from build123d import *

# Parameters (mm, degrees)
SKETCH1_W      = 6.35
SKETCH1_H      = 3.175
SKETCH1_W_2    = 12.7
SKETCH1_H_2    = 25
EXTRUDE1_DEPTH = 6.35


with BuildPart() as part:
    # Sketch1 → Extrude1 (new body)
    with BuildSketch(Plane.XY):
        with BuildLine():
            Line((-155, 0), (-155, 4))
            Line((-155, 4), (-180, 4))
            Line((-180, 4), (-180, 0))
            Line((-180, 0), (-195, 0))
            Line((-195, 0), (-179.241666667, 60))
            Line((-179.241666667, 60), (-146.84375, 60))
            Line((-146.84375, 60), (-146.84375, 85))
            Line((-146.84375, 85), (-172.675694444, 85))
            Line((-172.675694444, 85), (-166.109722222, 110))
            Line((-166.109722222, 110), (-146.84375, 110))
            Line((-146.84375, 110), (-146.84375, 135))
            Line((-146.84375, 135), (-159.54375, 135))
            Line((-159.54375, 135), (-152.977777778, 160))
            Line((-152.977777778, 160), (-134.14375, 160))
            ThreePointArc((-134.14375, 160), (-129.14375, 155), (-124.14375, 160))
            Line((-124.14375, 160), (-124.14375, 135))
            Line((-124.14375, 135), (-111.44375, 135))
            Line((-111.44375, 135), (-111.44375, 160))
            Line((-111.44375, 160), (0, 160))
            Line((0, 160), (124.14375, 160))
            ThreePointArc((124.14375, 160), (129.14375, 155), (134.14375, 160))
            Line((134.14375, 160), (152.977777778, 160))
            Line((152.977777778, 160), (159.54375, 135))
            Line((159.54375, 135), (111.44375, 135))
            Line((111.44375, 135), (111.44375, 110))
            Line((111.44375, 110), (166.109722222, 110))
            Line((166.109722222, 110), (172.675694444, 85))
            Line((172.675694444, 85), (111.44375, 85))
            Line((111.44375, 85), (111.44375, 60))
            Line((111.44375, 60), (179.241666667, 60))
            Line((179.241666667, 60), (195, 0))
            Line((195, 0), (180, 0))
            Line((180, 0), (180, 4))
            Line((180, 4), (155, 4))
            Line((155, 4), (155, 0))
            Line((155, 0), (-111.44375, 0))
            Line((-111.44375, 0), (-111.44375, 60))
            Line((-111.44375, 60), (-124.14375, 60))
            Line((-124.14375, 60), (-124.14375, 0))
            Line((-124.14375, 0), (-155, 0))
        make_face()
        with Locations((-53.175, 143.4125)):
            Rectangle(SKETCH1_W, SKETCH1_H, mode=Mode.SUBTRACT)
        with Locations((-117.79375, 97.5)):
            Rectangle(SKETCH1_W_2, SKETCH1_H_2, mode=Mode.SUBTRACT)
        with Locations((53.175, 143.4125)):
            Rectangle(SKETCH1_W, SKETCH1_H, mode=Mode.SUBTRACT)
    extrude(amount=EXTRUDE1_DEPTH)


solid = part.part
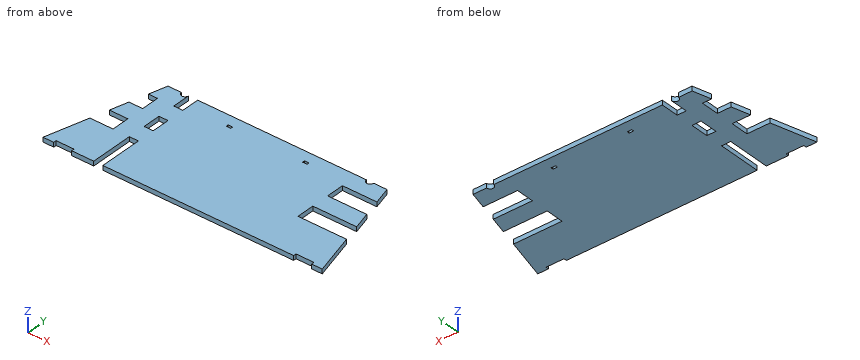
Could you check a few things on this model? Use its own coordinates, in mm. Coordinates: 2 decimals unless noted, no trailing zeros. Order: outer loops, then holes, each group sorted by start corner. A loop starts at its lowest first (then second) coordinate and runs counter-clockwise, first axis right, second up. Notation, with made-up numbers: (10, -35) -> (29, -35) arc R21 cw to (29, 2) -> close; hole circle Ø1 at (60, 46). An arc over 180 degrees is marked (long way). One line per item, written item: value. Start each with the question number.
1) Imagine slicing it at D-D on y = 67. List the corners of the cut face in (x, z) for me, plus the area to 3 significant figures.
2) I'm going to push flat-ended pins straight in: pin 1 (1.9 mm diameter, centred on x = -120.5, z = 3.5, fed in from +Y); pin 2 (1.9 mm diameter, centred on x = -53.5, z = 3, fed in from -Y); pin 3 (1.9 mm diameter, centred on x = -119, z = 4, fed in from -Y); pin 4 (1.2 mm diameter, centred on y = 2.5, z = 3.5, fed in from +X). Where does each tip first touch, or does it pass through?
3) If I drill on L1, parallel to Y at x = 148, z = 3.75; L2, parallel to Y at x = -51.5, z = 2 (3 decimals); L3, parallel to X at y = 144, z = 1.5, over which ranges is the centre line in solid material (lowest first)? Write a range as [from, to].
4) Imagine slicing it at C-C on z = 4. Count the separate pieces of the cut face and the enclosed holes in it, plus the area to 3 significant figures.
5) Imagine slicing it at A-A on y = 99. List the corners of the cut face in (x, z) for me.
6) Imagine slicing it at B-B on y = 15.5. List the corners of the cut face in (x, z) for me.
Answer list:
1. outline: (-146.84, 0) -> (111.44, 0) -> (111.44, 6.35) -> (-146.84, 6.35) -> close
1. area: 1,640 mm2
2. pin 1: stops at y = 135
2. pin 2: stops at y = 0
2. pin 3: stops at y = 60
2. pin 4: stops at x = 194.5
3. L1: y = [0, 60], [85, 110], [135, 160]
3. L2: y = [0, 141.825], [145, 160]
3. L3: x = [-157.18, -124.14], [-111.44, -56.35], [-50, 50], [56.35, 157.18]
4. separate pieces: 1
4. enclosed holes: 3
4. area: 49,900 mm2
5. outline: (-169, 0) -> (-124.14, 0) -> (-124.14, 6.35) -> (-169, 6.35) -> close; (-111.44, 0) -> (169, 0) -> (169, 6.35) -> (-111.44, 6.35) -> close
6. outline: (-190.93, 0) -> (-124.14, 0) -> (-124.14, 6.35) -> (-190.93, 6.35) -> close; (-111.44, 0) -> (190.93, 0) -> (190.93, 6.35) -> (-111.44, 6.35) -> close
